For this review, take the finished solid that the model builds, in its own axes (mm). Give positions to 0.01 mm unless a question says otherwise; leave off trailing zeros. Order: outer loops, then holes, each group sorted by start corner. A loop starts at its lowest first (then second) coordinate and runs counter-clockwise, first axis right, second up.
Item 1: Consider section B-B (x = 15.5). Give the boundary of the cut face in (y, z), plus the area to 3 significant figures.
Item 2: Consider section D-D (z = 1.3). Give the boundary of the cut face in (x, y), plus the area to 3 significant figures.
Item 3: For probe 1 along Y at (x, z) = (-15.5, 1.4); probe 2 along X at (y, z) = (35, 3.25); probe 3 along Y at (x, z) = (0, 2.9), list the stretches that pass through material, from the lowest coordinate up.
Item 4: Consider section C-C (y = 17). Give the boundary of the cut face in (x, z), plus the area to 3 significant figures.
Item 5: For P1, Ø2, axis at y = 9, z = 2, coming from the +X side; P2, Ø2, axis at y = 30.5, z = 2, coming from the -X side, all flat-tipped, find the tip position at first contact; note any pin that passes through.
Item 6: Consider section A-A (x = 0). Give the boundary of the cut face in (y, z), plus the area to 3 significant figures.
Autodesk Inventor part; units mm, degrees
ref_plane "YZ Plane" through (0, 0, 0) normal (1, 0, 0) x (0, 1, 0)
ref_plane "XZ Plane" through (0, 0, 0) normal (0, 1, 0) x (-1, 0, 0)
ref_plane "XY Plane" through (0, 0, 0) normal (0, 0, 1) x (1, 0, 0)
sketch "Sketch1" plane through (0, 0, 0) normal (0, 0, 1) x (1, 0, 0)
  line L0 (20, 35.0868) -> (15.0858, 40.001) construction
  line L1 (15.0858, 40.001) -> (-15.0858, 40.001) construction
  line L2 (-15.0858, 40.001) -> (-20, 35.0868) construction
  line L3 (-20, 35.0868) -> (-20, 4.9152) construction
  line L4 (-20, 4.9152) -> (-15.0858, 0.001) construction
  line L5 (-15.0858, 0.001) -> (15.0858, 0.001) construction
  line L6 (15.0858, 0.001) -> (20, 4.9152) construction
  line L7 (20, 4.9152) -> (20, 35.0868) construction
  spline S0 degree 3 number of poles 98 construction
  spline S1 degree 3 number of poles 98 construction
  spline S2 degree 3 number of poles 98 construction
  spline S3 degree 3 number of poles 98 construction
  circle A0 centre (0, 20.001) radius 11 construction
  spline S4 degree 3 number of poles 98 construction
  spline S5 degree 3 number of poles 98 construction
  spline S6 degree 3 number of poles 98 construction
  spline S7 degree 3 number of poles 98 construction
  line L8 (-152.3368, 49.5885) -> (152.3133, 49.5884) construction
  line L9 (-40.8871, 0.001) -> (40.8871, 0.001)
  line L10 (40.8871, 0.001) -> (40.8871, 40.001)
  line L11 (40.8871, 40.001) -> (-40.8871, 40.001)
  line L12 (-40.8871, 40.001) -> (-40.8871, 0.001)
  line L13 (-40.8871, 0.001) -> (40.8871, 40.001) construction
  line L14 (40.8871, 0.001) -> (-40.8871, 40.001) construction
  line L15 (40.8871, 40.001) -> (-40.8871, 40.001)
  line L16 (-40.8871, 40.001) -> (-40.8871, 49.5885)
  line L17 (-40.8871, 49.5885) -> (40.8871, 49.5885)
  line L18 (40.8871, 49.5885) -> (40.8871, 40.001)
  circle A1 centre (15.5, 4.501) radius 1.5
  circle A2 centre (-15.5, 4.501) radius 1.5
  circle A3 centre (-15.5, 35.501) radius 1.5
  circle A4 centre (15.5, 35.501) radius 1.5
  circle A5 centre (0, 20.001) radius 12.0934
  point P0 (0, 0)
extrude "Extrusion1" add sketch "Sketch1" along normal blind 4
sketch "Sketch2" plane through (0, 0, 4) normal (0, 0, 1) x (1, 0, 0)
  line L0 (36.8871, 28.0768) -> (36.8871, 34.0768) construction
  line L1 (36.8871, 28.0768) -> (40.8871, 28.0768) construction
  line L2 (40.8871, 34.0768) -> (40.8871, 28.0768) construction
  line L3 (36.8871, 34.0768) -> (40.8871, 34.0768) construction
  line L4 (36.8871, 6.8768) -> (36.8871, 12.8768) construction
  line L5 (36.8871, 6.8768) -> (40.8871, 6.8768) construction
  line L6 (40.8871, 12.8768) -> (40.8871, 6.8768) construction
  line L7 (36.8871, 12.8768) -> (40.8871, 12.8768) construction
  line L8 (-40.8871, 28.0768) -> (-40.8871, 34.0768) construction
  line L9 (-40.8871, 28.0768) -> (-36.8871, 28.0768) construction
  line L10 (-36.8871, 34.0768) -> (-36.8871, 28.0768) construction
  line L11 (-40.8871, 34.0768) -> (-36.8871, 34.0768) construction
  line L12 (-40.8871, 6.8768) -> (-40.8871, 12.8768) construction
  line L13 (-40.8871, 6.8768) -> (-36.8871, 6.8768) construction
  line L14 (-36.8871, 12.8768) -> (-36.8871, 6.8768) construction
  line L15 (-40.8871, 12.8768) -> (-36.8871, 12.8768) construction
  line L16 (-40.8871, 18.9768) -> (-40.8871, 21.9768) construction
  line L17 (-40.8871, 18.9768) -> (-36.8871, 18.9768) construction
  line L18 (-36.8871, 21.9768) -> (-36.8871, 18.9768) construction
  line L19 (-40.8871, 21.9768) -> (-36.8871, 21.9768) construction
  line L20 (36.8871, 18.9768) -> (36.8871, 21.9768) construction
  line L21 (36.8871, 18.9768) -> (40.8871, 18.9768) construction
  line L22 (40.8871, 21.9768) -> (40.8871, 18.9768) construction
  line L23 (36.8871, 21.9768) -> (40.8871, 21.9768) construction
  circle A0 centre (-38.8871, 20.4768) radius 1.6
  circle A1 centre (38.8871, 20.4768) radius 1.6
  line L24 (-36.6871, 34.2768) -> (-36.6871, 27.8768)
  line L25 (-36.6871, 27.8768) -> (-41.0871, 27.8768)
  line L26 (-41.0871, 27.8768) -> (-41.0871, 34.2768)
  line L27 (-41.0871, 34.2768) -> (-36.6871, 34.2768)
  line L28 (-36.6871, 13.0768) -> (-36.6871, 6.6768)
  line L29 (-36.6871, 6.6768) -> (-41.0871, 6.6768)
  line L30 (-41.0871, 6.6768) -> (-41.0871, 13.0768)
  line L31 (-41.0871, 13.0768) -> (-36.6871, 13.0768)
  line L32 (41.0871, 34.2768) -> (41.0871, 27.8768)
  line L33 (41.0871, 27.8768) -> (36.6871, 27.8768)
  line L34 (36.6871, 27.8768) -> (36.6871, 34.2768)
  line L35 (36.6871, 34.2768) -> (41.0871, 34.2768)
  line L36 (41.0871, 13.0768) -> (41.0871, 6.6768)
  line L37 (41.0871, 6.6768) -> (36.6871, 6.6768)
  line L38 (36.6871, 6.6768) -> (36.6871, 13.0768)
  line L39 (36.6871, 13.0768) -> (41.0871, 13.0768)
  point P0 (0, 0)
  dimension "d2" = 3.2
  dimension "d3" = 3.2
  dimension "d4" = 0.2
  dimension "d5" = 0.2
  dimension "d6" = 0.2
  dimension "d7" = 0.2
extrude "Extrusion2" cut sketch "Sketch2" against normal through all
sketch "Sketch3" plane through (0, 0, 4) normal (0, 0, 1) x (1, 0, 0)
  point P0 (0, 0)
properties part number "Motor_brace_2"
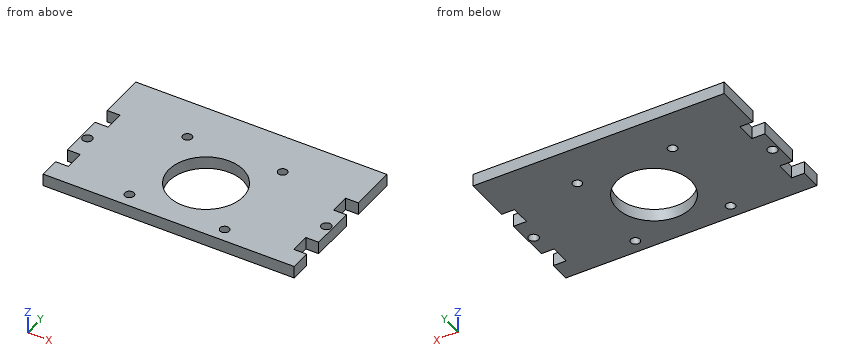
Resolved:
1. outline: (0, 0) - (3, 0) - (3, 4) - (0, 4) - close; (6, 0) - (34, 0) - (34, 4) - (6, 4) - close; (37, 0) - (49.59, 0) - (49.59, 4) - (37, 4) - close
1. area: 174 mm2
2. outline: (-40.89, 0) - (40.89, 0) - (40.89, 6.68) - (36.69, 6.68) - (36.69, 13.08) - (40.89, 13.08) - (40.89, 27.88) - (36.69, 27.88) - (36.69, 34.28) - (40.89, 34.28) - (40.89, 49.59) - (-40.89, 49.59) - (-40.89, 34.28) - (-36.69, 34.28) - (-36.69, 27.88) - (-40.89, 27.88) - (-40.89, 13.08) - (-36.69, 13.08) - (-36.69, 6.68) - (-40.89, 6.68) - close; hole circle Ø3.2 at (-38.89, 20.48); hole circle Ø3 at (-15.5, 4.5); hole circle Ø3 at (-15.5, 35.5); hole circle Ø24.19 at (0, 20); hole circle Ø3 at (15.5, 4.5); hole circle Ø3 at (15.5, 35.5); hole circle Ø3.2 at (38.89, 20.48)
2. area: 3,440 mm2
3. probe 1: y = 0 to 3, 6 to 34, 37 to 49.59
3. probe 2: x = -40.89 to -16.91, -14.09 to 14.09, 16.91 to 40.89
3. probe 3: y = 0 to 7.91, 32.09 to 49.59
4. outline: (-40.89, 0) - (-11.72, 0) - (-11.72, 4) - (-40.89, 4) - close; (11.72, 0) - (40.89, 0) - (40.89, 4) - (11.72, 4) - close
4. area: 233 mm2
5. P1: stops at x = 36.69
5. P2: stops at x = -36.69
6. outline: (0, 0) - (7.91, 0) - (7.91, 4) - (0, 4) - close; (32.09, 0) - (49.59, 0) - (49.59, 4) - (32.09, 4) - close
6. area: 102 mm2
